Here's how the part is built. I have some questions about the finished solid (model axes, mm). Face numbers are marked on the shaded views. A direction names the side the tool comes from. Coordinates: 2 decimals unless noted, no trailing zeros. Write each loop counter-clockwise with the first axis right and the second up, starting at its lowest first coordinate (ties: lowest second). Pieces come first, ordered by that corner, then holes.
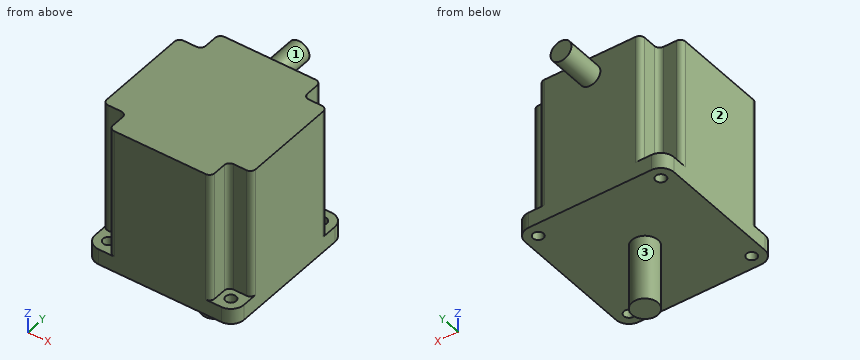
```python
from build123d import *

# Parameters (mm, degrees)
EXTRUDE_1_DEPTH     = 56
CUT_EXTRUDE_START   = -50
CUT_EXTRUDE_1_DEPTH = 50
FILLET_1_R          = 2
SKETCH_3_R          = 2
CUT_EXTRUDE_2_DEPTH = 65.222270281
SKETCH_4_R          = 5
EXTRUDE_2_DEPTH     = 25
SKETCH_5_R          = 4
EXTRUDE_3_DEPTH     = 15


with BuildPart() as part:
    # 草图1 → 凸台-拉伸1 (new body)
    with BuildSketch(Plane.XY):
        with BuildLine():
            Line((-23.5, 28.5), (23.5, 28.5))
            ThreePointArc((23.5, 28.5), (27.035533906, 27.035533906), (28.5, 23.5))
            Line((28.5, 23.5), (28.5, -23.5))
            ThreePointArc((28.5, -23.5), (27.035533906, -27.035533906), (23.5, -28.5))
            Line((23.5, -28.5), (-23.5, -28.5))
            ThreePointArc((-23.5, -28.5), (-27.035533906, -27.035533906), (-28.5, -23.5))
            Line((-28.5, -23.5), (-28.5, 23.5))
            ThreePointArc((-28.5, 23.5), (-27.035533906, 27.035533906), (-23.5, 28.5))
        make_face()
    extrude(amount=EXTRUDE_1_DEPTH)

    # 草图2 → 切除-拉伸1 (cut)
    with BuildSketch(Plane.XY.offset(56).offset(CUT_EXTRUDE_START)):
        with BuildLine():
            Line((-28.5, -19.5), (-19.5, -19.5))
            Line((-19.5, -19.5), (-19.5, -28.5))
            Line((-19.5, -28.5), (-23.5, -28.5))
            ThreePointArc((-23.5, -28.5), (-27.035533906, -27.035533906), (-28.5, -23.5))
            Line((-28.5, -23.5), (-28.5, -19.5))
        make_face()
        with BuildLine():
            Line((-28.5, 19.5), (-19.5, 19.5))
            Line((-19.5, 19.5), (-19.5, 28.5))
            Line((-19.5, 28.5), (-23.5, 28.5))
            ThreePointArc((-23.5, 28.5), (-27.035533906, 27.035533906), (-28.5, 23.5))
            Line((-28.5, 23.5), (-28.5, 19.5))
        make_face()
        with BuildLine():
            Line((23.5, 28.5), (19.5, 28.5))
            Line((19.5, 28.5), (19.5, 19.5))
            Line((19.5, 19.5), (28.5, 19.5))
            Line((28.5, 19.5), (28.5, 23.5))
            ThreePointArc((28.5, 23.5), (27.035533906, 27.035533906), (23.5, 28.5))
        make_face()
        with BuildLine():
            Line((28.5, -23.5), (28.5, -19.5))
            Line((28.5, -19.5), (19.5, -19.5))
            Line((19.5, -19.5), (19.5, -28.5))
            Line((19.5, -28.5), (23.5, -28.5))
            ThreePointArc((23.5, -28.5), (27.035533906, -27.035533906), (28.5, -23.5))
        make_face()
    extrude(amount=CUT_EXTRUDE_1_DEPTH, mode=Mode.SUBTRACT)

    # 圆角1
    fillet_1_edges = [part.edges().sort_by_distance(p)[0] for p in [
        (19.5, -28.5, 31),
        (19.5, -19.5, 31),
        (28.5, -19.5, 31),
        (-19.5, 28.5, 31),
        (-19.5, 19.5, 31),
        (-28.5, 19.5, 31),
        (28.5, 19.5, 31),
        (19.5, 19.5, 31),
        (19.5, 28.5, 31),
        (-28.5, -19.5, 31),
        (-19.5, -19.5, 31),
        (-19.5, -28.5, 31),
    ]]
    fillet(fillet_1_edges, radius=FILLET_1_R)

    # 草图3 → 切除-拉伸2 (cut, through all)
    with BuildSketch(Plane.XY.offset(6)):
        with Locations((-23.5, -23.5)):
            Circle(SKETCH_3_R)
        with Locations((-23.5, 23.5)):
            Circle(SKETCH_3_R)
        with Locations((23.5, 23.5)):
            Circle(SKETCH_3_R)
        with Locations((23.5, -23.5)):
            Circle(SKETCH_3_R)
    extrude(amount=-CUT_EXTRUDE_2_DEPTH, mode=Mode.SUBTRACT)

    # 草图4 → 凸台-拉伸2 (add)
    with BuildSketch(Plane(origin=(0, 0, 0), x_dir=(-1, 0, 0), z_dir=(0, 0, -1))):
        with Locations(Location((0, 0, 0), (0, 0, 180))):
            Circle(SKETCH_4_R)
    extrude(amount=EXTRUDE_2_DEPTH)

    # 草图5 → 凸台-拉伸3 (add)
    with BuildSketch(Plane(origin=(0, 28.5, 0), x_dir=(1, 0, 0), z_dir=(0, 1, 0))):
        with Locations((0, -49)):
            Circle(SKETCH_5_R)
    extrude(amount=EXTRUDE_3_DEPTH)


solid = part.part
```
1) Imagine slicing it at D-D on z = 22.5. Please give me the cut outline in (x, y), then the cut area to 3 significant figures.
Values follow:
outline: (-28.5, -17.5) arc R2 ccw to (-26.5, -19.5) - (-21.5, -19.5) arc R2 cw to (-19.5, -21.5) - (-19.5, -26.5) arc R2 ccw to (-17.5, -28.5) - (17.5, -28.5) arc R2 ccw to (19.5, -26.5) - (19.5, -21.5) arc R2 cw to (21.5, -19.5) - (26.5, -19.5) arc R2 ccw to (28.5, -17.5) - (28.5, 17.5) arc R2 ccw to (26.5, 19.5) - (21.5, 19.5) arc R2 cw to (19.5, 21.5) - (19.5, 26.5) arc R2 ccw to (17.5, 28.5) - (-17.5, 28.5) arc R2 ccw to (-19.5, 26.5) - (-19.5, 21.5) arc R2 cw to (-21.5, 19.5) - (-26.5, 19.5) arc R2 ccw to (-28.5, 17.5) - close
area: 2,920 mm2
2) I need wall thicknesses on probe 1 along Y at (x, z) = (23.5, 1.85); probe 2 along X at (y, z) = (-23, 2). Which ranges of each line are inside material? Lowest first, please.
Values follow:
probe 1: y = -28.5 to -25.5, -21.5 to 21.5, 25.5 to 28.5
probe 2: x = -28.5 to -25.44, -21.56 to 21.56, 25.44 to 28.5
3) Imagine slicing it at C-C on x = 0. Please give me the cut outline in (y, z), then the cut area to 3 significant figures.
Values follow:
outline: (-28.5, 0) - (-5, 0) - (-5, -25) - (5, -25) - (5, 0) - (28.5, 0) - (28.5, 45) - (43.5, 45) - (43.5, 53) - (28.5, 53) - (28.5, 56) - (-28.5, 56) - close
area: 3,560 mm2
4) On a 3-axis mill with a long thin cutter (end or side, diameter ignored), from which of +Z, -Z, +X, -X, +Y, -Y can I reach the whole of each face in a straight line? I mean the marked faces 1, 2 and 3. Say none if no direction works.
Values follow:
face 1: +Y
face 2: +Z, -Z, -X, +Y, -Y
face 3: -Z
5) Imagine slicing it at A-A on z = 3. Please give me the cut outline in (x, y), then the cut area to 3 significant figures.
Values follow:
outline: (-28.5, -23.5) arc R5 ccw to (-23.5, -28.5) - (23.5, -28.5) arc R5 ccw to (28.5, -23.5) - (28.5, 23.5) arc R5 ccw to (23.5, 28.5) - (-23.5, 28.5) arc R5 ccw to (-28.5, 23.5) - close; hole circle Ø4 at (-23.5, -23.5); hole circle Ø4 at (-23.5, 23.5); hole circle Ø4 at (23.5, -23.5); hole circle Ø4 at (23.5, 23.5)
area: 3,180 mm2
6) Will these pins go through, and if not, where does the flat tip stop? pin 1 (1.5 mm diameter, centred on y = 27.5, z = 6.5, fed in from -X); pin 2 (3.5 mm diameter, centred on x = -21.5, y = -23, fed in from +Z); pin 3 (3 mm diameter, centred on x = -23.5, y = 23.5, fed in from -Z); pin 4 (5.5 mm diameter, centred on x = 23.5, z = 32.5, fed in from -Y).
Values follow:
pin 1: stops at x = -27.13
pin 2: stops at z = 6
pin 3: passes through
pin 4: stops at y = -19.65
7) Imagine slicing it at B-B on y = 0. Please give me the cut outline in (x, z), then the cut area to 3 significant figures.
Values follow:
outline: (-28.5, 0) - (-5, 0) - (-5, -25) - (5, -25) - (5, 0) - (28.5, 0) - (28.5, 56) - (-28.5, 56) - close
area: 3,440 mm2
